Source: three-view drawing plus pictorial views. Frame: mm from the lowest corner of the part. A direction names the side the tool comes from. Give positions to 0.01 mm unless a question says otherwise; leave off trailing zeros. Loops run counter-clockwise (first coordinate to the right, second up) from the corner with the lowest first, then second, coordinate; pieces in that order, holes last. Notation, with made-up numbers: M 25.25,-38.5 L 52.25,-38.5 A21 ccw 52.25,-0.5 Z; hole C 27.25,-2 d2. An arc over 180 degrees is marked long. Answer as a JSON object with one key per item and string values. Group by question number.
1) Access query for the marked faces 1, 2 and 3. Directions: +Z, -Z, +X, -X, +Y, -Y. A direction counts if a zero-diameter tool reaches every point of the face in a straight line with its end or side. Return the directions, or none.
2) Section query C-C on x = 22.75. Return loops of the section in (y, z).
3) Section query A-A on x = 28. Return loops of the section in (y, z).
4) Section query D-D on z = 20.25. Return loops of the section in (x, y).
5) Section query B-B on z = 28. Return loops of the section in (x, y).
6) Ray query, L1, parallel to X at y = 4.8, z = 2; L2, parallel to X at y = 2.5, z = 17.5. Return the intervals inside material, ascending.
7) First-contact query: P1, Ø1.2, axis at x = 16, y = 2, coming from the -Z side; P2, Ø2.5, axis at x = 28, z = 2, coming from the +Y side; P3, Ø1.2, axis at y = 2, z = 14.5, coming from the +X side; P4, Ø1.2, axis at x = 2, z = 28, coming from the -Y side. Flat tips, straight axial feed; report the tip coordinate or a pass-through.
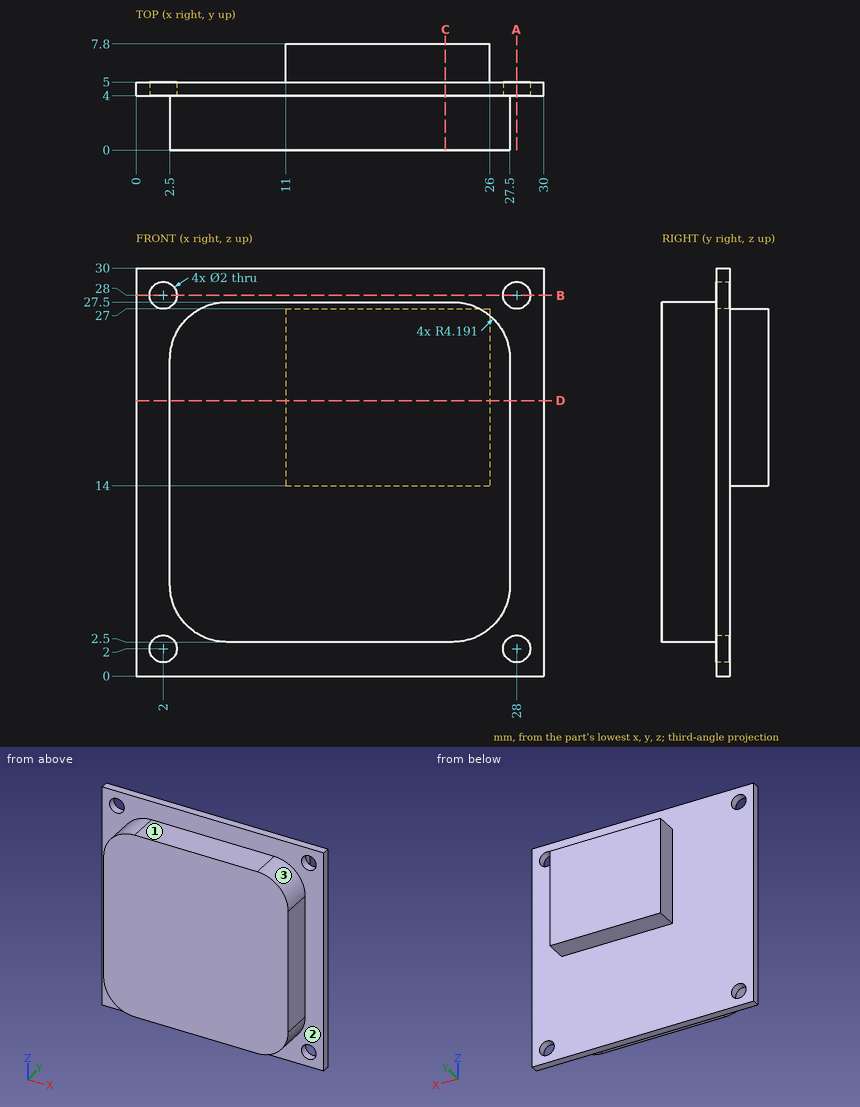
Output:
{
 "1": {"face 1": "+Z, +X, -X, -Y", "face 2": "-Y", "face 3": "+Z, +X, -Y"},
 "2": {"outline": "M 0,2.5 L 4,2.5 L 4,0 L 5,0 L 5,14 L 7.8,14 L 7.8,27 L 5,27 L 5,30 L 4,30 L 4,27.5 L 0,27.5 Z"},
 "3": {"outline": "M 4,0 L 5,0 L 5,1 L 4,1 Z; M 4,3 L 5,3 L 5,27 L 4,27 Z; M 4,29 L 5,29 L 5,30 L 4,30 Z"},
 "4": {"outline": "M 0,4 L 2.5,4 L 2.5,0 L 27.5,0 L 27.5,4 L 30,4 L 30,5 L 26,5 L 26,7.8 L 11,7.8 L 11,5 L 0,5 Z"},
 "5": {"outline": "M 0,4 L 1,4 L 1,5 L 0,5 Z; M 3,4 L 27,4 L 27,5 L 3,5 Z; M 29,4 L 30,4 L 30,5 L 29,5 Z"},
 "6": {"L1": "x = 0 to 1, 3 to 27, 29 to 30", "L2": "x = 2.5 to 27.5"},
 "7": {"P1": "stops at z = 2.5", "P2": "stops at y = 5", "P3": "stops at x = 27.5", "P4": "passes through"}
}
